```python
from build123d import *

# Parameters (mm, degrees)
F0_W          = 13.3
F0_H          = 13.3
F0_W_2        = 10.3
F0_H_2        = 10.3
F1_DEPTH      = 20
F2_DEPTH      = 1.5
F3_W          = 4
F3_H          = 13.3
F3_W_2        = 5.3
F4_DEPTH      = 25
F5_T1_DEPTH   = 46.6
F6_R          = 1.975
F7_DEPTH      = 25
F7_DEPTH_BACK = 25


# Not quite as in the source:
# - a fillet or chamfer that OpenCascade refuses, or shapes differently, is made with other operations: its cross-section is extruded or revolved along the edge and cut away or added


with BuildPart() as f1:
    # F0 (on Top) → F1 (new body)
    with BuildSketch(Plane.XY):
        Rectangle(F0_W, F0_H)
        Rectangle(F0_W_2, F0_H_2, mode=Mode.SUBTRACT)
    extrude(amount=-F1_DEPTH)

    # F0 (on Top) → F2 (join)
    with BuildSketch(Plane.XY):
        Rectangle(F0_W, F0_H)
        Rectangle(F0_W_2, F0_H_2, mode=Mode.SUBTRACT)
        Rectangle(F0_W_2, F0_H_2)
    extrude(amount=F2_DEPTH)

    # F3 (on face) → F4 (join)
    with BuildSketch(Plane.XY.offset(1.5)):
        with Locations((-4.65, 0)):
            Rectangle(F3_W, F3_H)
        with Locations((4.65, 0)):
            Rectangle(F3_W, F3_H)
        Rectangle(F3_W_2, F3_H)
    extrude(amount=F4_DEPTH)

    # F5: fillet of radius 6.66 on 2 edges, made by hand

    # F5_s2 → F5_t1 (cut)
    with BuildSketch(Plane.YZ.offset(-23.3)):
        with BuildLine():
            ThreePointArc((-0.01, 26.5), (4.6993311627, 24.5493311627), (6.65, 19.84))
            Line((6.65, 19.84), (6.65, 26.5))
            Line((6.65, 26.5), (-0.01, 26.5))
        make_face()
        with BuildLine():
            ThreePointArc((-6.65, 19.84), (-4.6993311627, 24.5493311627), (0.01, 26.5))
            Line((0.01, 26.5), (-6.65, 26.5))
            Line((-6.65, 26.5), (-6.65, 19.84))
        make_face()
    extrude(amount=F5_T1_DEPTH, mode=Mode.SUBTRACT)

    # F6 (on face) → F7 (cut, two sides)
    with BuildSketch(Plane.YZ.offset(6.65)) as f7_sk:
        with Locations((0.01, 4)):
            Circle(F6_R)
        with Locations((0.01, 19.84)):
            Circle(F6_R)
    extrude(amount=-F7_DEPTH, mode=Mode.SUBTRACT)
    extrude(f7_sk.sketch, amount=F7_DEPTH_BACK, mode=Mode.SUBTRACT)


solid = f1.part
```
Can you work these out from the model? Positions are in its coordinate system, mm. A direction names the side the tool comes from. Round coordinates to 2 decimals unless told otherwise and drop trailing zeros. Order: outer loops, then holes, each group sorted by start corner. A loop starts at its lowest first (then second) coordinate and runs counter-clockwise, first axis right, second up. Notation, with made-up numbers: (25, 16.5) -> (65, 16.5) arc R27 cw to (65, 33.5) -> close; hole circle Ø9 at (-2, 83.5). An arc over 180 degrees is marked (long way). Return JSON: item names as keys, results as strings. Group by question number.
1. Will these pins go through, and if not, where does the flat tip stop? pin 1 (5 mm diameter, centred on x = 1, y = 0.5, fed in from -Z); pin 2 (3 mm diameter, centred on y = 0.01, z = 19.84, fed in from -X).
2. If we section it at D-D, the plane y = 1: Write out the boundary of the cut face in (x, z).
3. If we section it at C-C, the plane z = 4.5: Write out the boundary of the cut face in (x, y).
4. Which directions (+Z, -Z, +X, -X, +Y, -Y) give clear straight access to the entire face, cutting with the end or side of a thin tool? Please do faces 4 (the face through (-0.093, -4.754, 24.494)), 5 (the face through (0, -5.15, -10)).
5. We'd pull the mould along X, two halves only. Please class faces 1 (the face through (0, 5.15, -10)), 2 (the face through (6.65, -3, 3)), 3 (the face through (-6, 0, -20)): released by +X, released by -X, zero draft, split by the parting line, or undercut.
6. If we section it at B-B, the plane z = -17: Write out the boundary of the cut face in (x, y).
7. If we section it at A-A, the plane x = -2: Write out the boundary of the cut face in (y, z) (3 decimals).
8. I need wall thicknesses on line 1 (Z direction, x = -1.25, y = 0.01) (3 decimals); line 2 (X direction, y = 2.25, z = -18). Which ranges of each line are inside material? Lowest first, please. Write a range as [from, to].
Output values:
{
 "1": {"pin 1": "z = 0", "pin 2": "through"},
 "2": {"outline": "(-6.65, -20) -> (-5.15, -20) -> (-5.15, 0) -> (5.15, 0) -> (5.15, -20) -> (6.65, -20) -> (6.65, 2.29) -> (-6.65, 2.29) -> close; (-6.65, 5.71) -> (6.65, 5.71) -> (6.65, 18.13) -> (-6.65, 18.13) -> close; (-6.65, 21.55) -> (6.65, 21.55) -> (6.65, 26.42) -> (-6.65, 26.42) -> close"},
 "3": {"outline": "(-6.65, -6.65) -> (6.65, -6.65) -> (6.65, -1.9) -> (-6.65, -1.9) -> close; (-6.65, 1.92) -> (6.65, 1.92) -> (6.65, 6.65) -> (-6.65, 6.65) -> close"},
 "4": {"face 4": "+Z, +X, -X, -Y", "face 5": "-Z"},
 "5": {"face 1": "undercut", "face 2": "released by +X", "face 3": "zero draft"},
 "6": {"outline": "(-6.65, -6.65) -> (6.65, -6.65) -> (6.65, 6.65) -> (-6.65, 6.65) -> close; hole (-5.15, -5.15) -> (5.15, -5.15) -> (5.15, 5.15) -> (-5.15, 5.15) -> close"},
 "7": {"outline": "(-6.65, -20) -> (-5.15, -20) -> (-5.15, 0) -> (5.15, 0) -> (5.15, -20) -> (6.65, -20) -> (6.65, 19.84) arc R6.66 ccw to (0, 26.5) arc R6.66 ccw to (-6.65, 19.84) -> close; hole circle Ø3.95 at (0.01, 4); hole circle Ø3.95 at (0.01, 19.84)"},
 "8": {"line 1": "[0, 2.025], [5.975, 17.865], [21.815, 26.5]", "line 2": "[-6.65, -5.15], [5.15, 6.65]"}
}
